Check sheet for the modelled part. Datum: model origin and axes. Units: mm. A direction names the side the tool comes from. Coordinates: 2 decimals unless noted, no trailing zeros. Order: outer loops, then holes, each group sorted by start corner. A loop starts at its lowest first (then second) coordinate and runs counter-clockwise, first axis right, second up.
1. Draft check along Y on faces 1 (the cylindrical face through (110.545, 12.579, 4.624)), 2 (the flat face through (0, 16, 3)), 3 (the flat face through (74, 31.75, 3)). Enter one of: released by +Y, released by -Y, zero draft, split by the parting line, or undercut.
2. Thickness scan on line 1 (Y direction, x = 114.3, z = 2.2); line 2 (Y direction, x = 114.3, z = 4.15); line 3 (X direction, y = 21.5, z = 5.75). Record the ranges inside material, lowest first.
3. Gauge pin test, flat end, axial feed: pin 1 Ø5 at (x, y) = (107, 19.5) entering from +Z. Record the tip position at first contact, or that the pin passes through.
4. Set-up check for faces 4 (the cylindrical face through (119.794, 18.961, 1.453)), 5 (the cylindrical face through (118.006, 20.299, 4.624)): record each of +Z, -Z, +X, -X, +Y, -Y from which the full face is reachable in a straight line by a thin tool's end or side.
5. Cross-section at B-B (z = 1). Count the separate pieces of the cut face and the enclosed holes in it, then the cut area to 3 significant figures.
6. Cross-section at A-A (x = 114.3). Enter the section's corners in (y, z), then the cut area to 3 significant figures.
Autodesk Inventor part; units mm, degrees
ref_plane "YZ Plane" through (0, 0, 0) normal (1, 0, 0) x (0, 1, 0)
ref_plane "XZ Plane" through (0, 0, 0) normal (0, 1, 0) x (-1, 0, 0)
ref_plane "XY Plane" through (0, 0, 0) normal (0, 0, 1) x (1, 0, 0)
sketch "Sketch1" plane through (0, 0, 0) normal (0, 0, 1) x (1, 0, 0)
  line L0 (0, 0) -> (146.05, 0)
  line L1 (146.05, 0) -> (146.05, 31.75)
  line L2 (146.05, 31.75) -> (0, 31.75)
  line L3 (0, 31.75) -> (0, 0)
  dimension "d0" = 146.05
  dimension "d1" = 31.75
extrude "Extrusion1" add sketch "Sketch1" along normal blind 6.35
sketch "Sketch2" plane through (0, 0, 6.35) normal (0, 0, 1) x (1, 0, 0)
  line L0 (146.05, 0) -> (146.05, 31.75)
  line L1 (146.05, 12.7901) -> (163.1696, 12.7901) construction
  line L2 (0, 0) -> (146.05, 0)
  line L3 (114.3, 0) -> (114.3, 15.875)
  line L4 (114.3, 0) -> (130.175, 0) construction
  circle A0 centre (114.3, 15.875) radius 8.001
  point P0 (114.3, 7.874)
  point P1 (121.2291, 11.8745)
  point P2 (121.2291, 19.8755)
  point P3 (114.3, 23.876)
  point P4 (107.3709, 19.8755)
  point P5 (107.3709, 11.8745)
  dimension "d9" = 16.002
  dimension "d7" = 90
  dimension "d17" = 31.75
  dimension "d48" = 360
  dimension "d79" = 31.75
  dimension "d80" = 15.875
  dimension "d81" = 15.875
hole "Hole2" at (114.3, 7.874, 6.35) at (121.2291, 11.8745, 6.35) at (121.2291, 19.8755, 6.35) at (114.3, 23.876, 6.35) at (107.3709, 19.8755, 6.35) at (107.3709, 11.8745, 6.35) direction (0, 0, -1) diameter 3.4036 end through all counterbore diameter 6.5024 counterbore depth 3.4036
hole "Hole3" at (114.3, 15.875, 6.35) direction (0, 0, -1) diameter 6.35 end through all
sketch "Sketch5" plane through (0, 0, 6.35) normal (0, 0, 1) x (1, 0, 0)
  line L0 (0, 31.75) -> (0, 0)
  line L1 (146.05, 31.75) -> (0, 31.75)
  circle A0 centre (114.3, 15.875) radius 3.175
  circle A1 centre (107.3709, 19.8755) radius 3.2512
  circle A2 centre (121.2291, 19.8755) radius 3.2512
  circle A3 centre (114.3, 7.874) radius 3.2512
  circle A4 centre (121.2291, 11.8745) radius 3.2512
  circle A5 centre (114.3, 23.876) radius 3.2512
  circle A6 centre (107.3709, 11.8745) radius 3.2512
  line L2 (0, 0) -> (146.05, 0)
  line L3 (146.05, 0) -> (146.05, 31.75)
  line L4 (146.05, 31.75) -> (0, 31.75)
  line L5 (0, 31.75) -> (0, 0)
  point P0 (9.525, 15.875)
  point P1 (136.525, 15.875)
  dimension "d64" = 31.75
  dimension "d65" = 15.875
  dimension "d68" = 15.875
  dimension "d69" = 9.525
  dimension "d71" = 9.525
hole "Hole4" at (9.525, 15.875, 6.35) at (136.525, 15.875, 6.35) direction (0, 0, -1) diameter 6.35 end through all
equation "\"d81\" = d80"
properties part number "core hex motor to 30x30 mount"
Data:
1. face 1: undercut
1. face 2: zero draft
1. face 3: released by +Y
2. line 1: y = 0 to 6.17, 9.58 to 12.7, 19.05 to 22.17, 25.58 to 31.75
2. line 2: y = 0 to 4.62, 11.13 to 12.7, 19.05 to 20.62, 27.13 to 31.75
2. line 3: x = 0 to 104.55, 110.19 to 112.08, 116.52 to 118.41, 124.05 to 146.05
3. pin 1: stops at z = 2.95
4. face 4: +Z, -Z
4. face 5: +Z
5. separate pieces: 1
5. enclosed holes: 9
5. area: 4,490 mm2
6. outline: (0, 0) - (6.17, 0) - (6.17, 2.95) - (4.62, 2.95) - (4.62, 6.35) - (0, 6.35) - close; (9.58, 0) - (12.7, 0) - (12.7, 6.35) - (11.13, 6.35) - (11.13, 2.95) - (9.58, 2.95) - close; (19.05, 0) - (22.17, 0) - (22.17, 2.95) - (20.62, 2.95) - (20.62, 6.35) - (19.05, 6.35) - close; (25.58, 0) - (31.75, 0) - (31.75, 6.35) - (27.13, 6.35) - (27.13, 2.95) - (25.58, 2.95) - close
6. area: 97.0 mm2
